Part model, mm, in its own coordinate system. Face numbers are marked on the shaded views. A direction names the side the tool comes from. Round coordinates to 2 decimals unless told otherwise and drop trailing zeros. Loops run counter-clockwise (first coordinate to the right, second up) from the corner with the lowest first, then second, coordinate; pieces in that order, holes last.
(1) Cut at C-C on y = -12. List the corners of the cut face in (x, z), then the cut area to 3 significant figures.
(2) Cut at B-B on x = 2.25. List the corners of the cut face in (y, z), then the cut area to 3 significant figures.
(3) Tool access for the marked faces 4 and 5: list every direction of +Z, -Z, +X, -X, +Y, -Y with a clear straight run to the whole face (end or side of a thin tool).
(4) Mould opens along Z. For the marked faces 1, 2 and 3 say: +Z half, -Z half, draft (parallel to the pull), parting line (faces both ways), or undercut.
(5) Probe probe 1 along X at (y, z) = (-0.75, 1.4); probe 2 along Y at (x, z) = (-11.25, 3.25); probe 3 along X at (y, z) = (-15, 0.25). List the from-to ranges inside material, lowest first.
(6) Flat gauge pins, fed straight in: pin 1 (2 mm diameter, centred on x = 3, z = 2, fed in from +Y); pin 2 (1.7 mm diameter, centred on x = -12, z = 2.5, fed in from -Y); pin 3 (1.7 mm diameter, centred on y = 0, z = 2.5, fed in from +X). Where does each tip first touch, or does it go through?
(7) Cut at A-A on z = 3.45. List the corners of the cut face in (x, y).
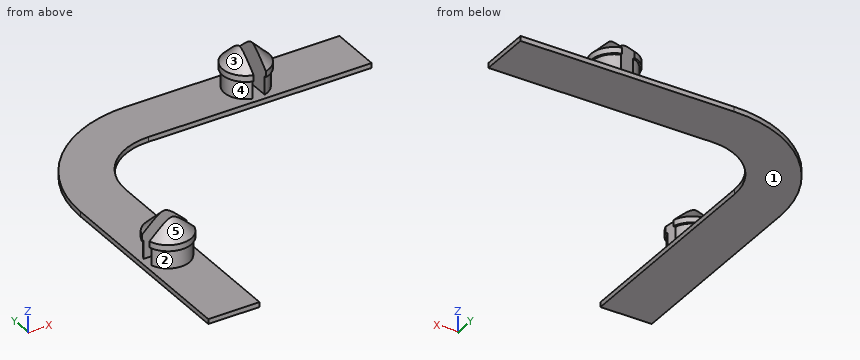
from build123d import *

# Parameters (mm, degrees)
SKICA2_W                 = 27.5
SKICA2_H                 = 4.2
P_IDAT_VYSUNUT_M2_DEPTH  = 0.4
SKICA3_R                 = 1.75
P_IDAT_VYSUNUT_M3_DEPTH  = 1.5
SKICA5_R                 = 1.9
P_IDAT_VYSUNUT_M5_DEPTH  = 2
ZKOSEN_2_SIZE            = 1.5
SKICA7_W                 = 1
SKICA7_H                 = 5
ODEBRAT_VYSUNUT_M1_DEPTH = 3.5
SKICA8_W                 = 4.2
SKICA8_H                 = 22.5
P_IDAT_VYSUNUT_M6_DEPTH  = 0.4
SKICA9_R                 = 1.75
P_IDAT_VYSUNUT_M7_DEPTH  = 1.5
SKICA10_R                = 1.9
P_IDAT_VYSUNUT_M8_DEPTH  = 2
ZKOSEN_3_SIZE            = 1.5
SKICA12_W                = 5
SKICA12_H                = 1
ODEBRAT_VYSUNUT_M2_DEPTH = 3.5
ZAOBLIT1_R               = 5
ZAOBLIT2_R               = 10


with BuildPart() as part:
    # Skica2 → Přidat vysunutím2 (new body)
    with BuildSketch(Plane.XY):
        Rectangle(SKICA2_W, SKICA2_H)
    extrude(amount=P_IDAT_VYSUNUT_M2_DEPTH)

    # Skica3 → Přidat vysunutím3 (add)
    with BuildSketch(Plane.XY.offset(0.4)):
        with Locations((4.75, 0)):
            Circle(SKICA3_R)
    extrude(amount=P_IDAT_VYSUNUT_M3_DEPTH)

    # Skica5 → Přidat vysunutím5 (add)
    with BuildSketch(Plane.XY.offset(1.9)):
        with Locations((4.75, 0)):
            Circle(SKICA5_R)
    extrude(amount=P_IDAT_VYSUNUT_M5_DEPTH)

    # Zkosení2
    zkosen_2_edges = [part.edges().sort_by_distance(p)[0] for p in [
        (2.85, 0, 3.9),
    ]]
    chamfer(zkosen_2_edges, length=ZKOSEN_2_SIZE)

    # Skica7 → Odebrat vysunutím1 (cut)
    with BuildSketch(Plane.XY.offset(3.9)):
        with Locations((4.75, 0)):
            Rectangle(SKICA7_W, SKICA7_H)
    extrude(amount=-ODEBRAT_VYSUNUT_M1_DEPTH, mode=Mode.SUBTRACT)

    # Skica8 → Přidat vysunutím6 (add)
    with BuildSketch(Plane(origin=(0, 0, 0), x_dir=(-1, 0, 0), z_dir=(0, 0, -1))):
        with Locations((11.65, -13.35)):
            Rectangle(SKICA8_W, SKICA8_H)
    extrude(amount=-P_IDAT_VYSUNUT_M6_DEPTH)

    # Skica9 → Přidat vysunutím7 (add)
    with BuildSketch(Plane.XY.offset(0.4)):
        with Locations((-11.65, -16)):
            Circle(SKICA9_R)
    extrude(amount=P_IDAT_VYSUNUT_M7_DEPTH)

    # Skica10 → Přidat vysunutím8 (add)
    with BuildSketch(Plane.XY.offset(1.9)):
        with Locations((-11.65, -16)):
            Circle(SKICA10_R)
    extrude(amount=P_IDAT_VYSUNUT_M8_DEPTH)

    # Zkosení3
    zkosen_3_edges = [part.edges().sort_by_distance(p)[0] for p in [
        (-13.55, -16, 3.9),
    ]]
    chamfer(zkosen_3_edges, length=ZKOSEN_3_SIZE)

    # Skica12 → Odebrat vysunutím2 (cut)
    with BuildSketch(Plane.XY.offset(3.9)):
        with Locations((-11.65, -16)):
            Rectangle(SKICA12_W, SKICA12_H)
    extrude(amount=-ODEBRAT_VYSUNUT_M2_DEPTH, mode=Mode.SUBTRACT)

    # Zaoblit1
    zaoblit1_edges = [part.edges().sort_by_distance(p)[0] for p in [
        (-9.55, -2.1, 0.2),
    ]]
    fillet(zaoblit1_edges, radius=ZAOBLIT1_R)

    # Zaoblit2
    zaoblit2_edges = [part.edges().sort_by_distance(p)[0] for p in [
        (-13.75, 2.1, 0.2),
    ]]
    fillet(zaoblit2_edges, radius=ZAOBLIT2_R)


solid = part.part
Final values:
1. outline: (-13.75, 0) - (-9.55, 0) - (-9.55, 0.4) - (-13.75, 0.4) - close
1. area: 1.68 mm2
2. outline: (-2.1, 0) - (2.1, 0) - (2.1, 0.4) - (-2.1, 0.4) - close
2. area: 1.68 mm2
3. face 4: -X
3. face 5: +Z, -Y
4. face 1: -Z half
4. face 2: undercut
4. face 3: +Z half
5. probe 1: x = 3.17 to 4.25, 5.25 to 6.33
5. probe 2: y = -16.97 to -16.5, -15.5 to -15.03
5. probe 3: x = -13.75 to -9.55
6. pin 1: stops at y = 1.75
6. pin 2: stops at y = -17.9
6. pin 3: stops at x = 6.65
7. outline: (-12.34, -16.5) arc R0.85 ccw to (-10.96, -16.5) - close; (-12.34, -15.5) - (-10.96, -15.5) arc R0.85 ccw to start; (4.25, -0.69) - (4.25, 0.69) arc R0.85 ccw to start; (5.25, -0.69) arc R0.85 ccw to (5.25, 0.69) - close
